Geometry: final body of the model. Coordinates: model frame, mm. A direction names the side the tool comes from. Coordinates: 2 decimals unless noted, no trailing zeros. Order: outer loops, then holes, each group sorted by start corner. A loop starts at its lowest first (then second) coordinate and runs counter-clockwise, first axis right, second up. Notation, with made-up numbers: (20, 72.25) -> (77, 72.25) arc R6 cw to (77, 77.25) -> close; hole circle Ø5 at (86.25, -0.75). An arc over 180 degrees is marked (long way). Answer in a Markdown table with one row per item. Add a question column.
1) Section query D-D on x = 7.5. Return the cut outline in (y, z).
2) Section query B-B on y = 29.5. Return the cut outline in (x, z).
3) Set-up query: faces 1 (the face through (12.7, 45, -43)), 2 (the face through (1, 13, 0)), 3 (the face through (-12.7, 45, -43)), 4 (the face through (1, 13, -101.6)). Return all of +Z, -Z, +X, -X, +Y, -Y with unobstructed straight access to the full face (end or side cutting, diameter ignored); none if empty.
4) Section query A-A on x = 22.5. Return the cut outline in (y, z).
5) Section query C-C on z = -19. Return the cut outline in (x, y), then the cut area to 3 significant figures.
6) Pull-direction query (Z, two-part tool) for faces 5 (the face through (-38.1, 32, -65)), 6 (the face through (-5.47, 127.15, -90.68)), 7 (the face through (3.72, 101.245, -119.34)); classes: +Z half, -Z half, draft (parallel to the pull), parting line (faces both ways), or undercut.
7) Contact query for flat-ended pins moving along their axis: P1, Ø10, axis at x = 25.5, y = 95, coming from the +Z side; P2, Ø10, axis at y = 84.5, z = -131, coming from the -X side; P3, Ø10, axis at x = -14.5, y = 14, coming from the -Z side. Output: stop coordinate, or through.
8) Ray query, line 1 (X direction, y = 38.5, z = -40); line 2 (Y direction, x = 24.5, z = -35); line 3 (X direction, y = 82, z = -121.5). Return the intervals inside material, ascending. Write a range as from..to.
```python
from build123d import *

# Parameters (mm, degrees)
BOSS_EXTRUDE1_DEPTH = 38.1
BOSS_EXTRUDE2_REACH = 114.341
SKETCH3_W           = 25.4
SKETCH3_H           = 88.161149917
SKETCH4_R           = 38.1
BOSS_EXTRUDE3_DEPTH = 76.2
SKETCH5_R           = 28.575
CUT_EXTRUDE1_DEPTH  = 76.2


with BuildPart() as part:
    # Sketch1 → Boss-Extrude1 (new body, symmetric)
    with BuildSketch(Plane(origin=(0, 0, 0), x_dir=(0, 0, -1), z_dir=(1, 0, 0))):
        Polygon((0, 0), (0, 25.4), (50.8, 25.4), (100.244555556, 80.313742191), (128.299578523, 55.052886048), (101.6, 25.4), (101.6, 0), align=None)
    extrude(amount=BOSS_EXTRUDE1_DEPTH, both=True)

    # Sketch3 → Boss-Extrude2 (add, up to next)
    with BuildSketch(Plane(origin=(0, 11.372488517, 12.630428071), x_dir=(1, 0, 0), z_dir=(0, 0.669130606, 0.743144825)), mode=Mode.PRIVATE) as boss_extrude2_sk1:
        with Locations((0, 62.956453526)):
            Rectangle(SKETCH3_W, SKETCH3_H)
    boss_extrude2_tool1 = extrude(boss_extrude2_sk1.sketch, amount=-BOSS_EXTRUDE2_REACH, mode=Mode.PRIVATE) - part.part
    add(boss_extrude2_tool1.solids().sort_by_distance((0, 58.158251, -29.495662))[0])

    # Sketch4 → Boss-Extrude3 (add)
    with BuildSketch(Plane(origin=(0, -39.149223768, -43.479617863), x_dir=(-1, 0, 0), z_dir=(0, -0.669130606, -0.743144825))):
        with Locations((0, 126.761442167)):
            Circle(SKETCH4_R)
    extrude(amount=-BOSS_EXTRUDE3_DEPTH)

    # Sketch5 → Cut-Extrude1 (cut)
    with BuildSketch(Plane(origin=(0, -39.149223768, -43.479617863), x_dir=(-1, 0, 0), z_dir=(0, -0.669130606, -0.743144825))):
        with Locations((0, 126.761442167)):
            Circle(SKETCH5_R)
    extrude(amount=-CUT_EXTRUDE1_DEPTH, mode=Mode.SUBTRACT)


solid = part.part
```
Result:
| question | item | result |
|---|---|---|
| 1 | outline | (0, -101.6) -> (25.4, -101.6) -> (34.56, -109.85) -> (85.55, -53.22) -> (78.28, -46.68) -> (77.81, -47.19) -> (25.4, 0) -> (0, 0) -> close; (75.54, -146.75) -> (82.81, -153.29) -> (133.8, -96.67) -> (126.53, -90.12) -> close |
| 2 | outline | (-38.1, -105.29) -> (38.1, -105.29) -> (38.1, -54.49) -> (12.7, -54.49) -> (12.7, -3.69) -> (-12.7, -3.69) -> (-12.7, -54.49) -> (-38.1, -54.49) -> close |
| 3 | face 1 | +Z, +X |
| 3 | face 2 | +Z, +X, -X, +Y, -Y |
| 3 | face 3 | +Z, -X |
| 3 | face 4 | -Z, +X, -X, -Y |
| 4 | outline | (0, -101.6) -> (25.4, -101.6) -> (41.96, -116.51) -> (92.95, -59.89) -> (83.19, -51.1) -> (57.46, -79.67) -> (25.4, -50.8) -> (25.4, 0) -> (0, 0) -> close; (68.14, -140.09) -> (77.9, -148.87) -> (128.89, -92.25) -> (119.13, -83.46) -> close |
| 5 | outline | (-38.1, 0) -> (38.1, 0) -> (38.1, 25.4) -> (12.7, 25.4) -> (12.7, 46.5) -> (-12.7, 46.5) -> (-12.7, 25.4) -> (-38.1, 25.4) -> close |
| 5 | area | 2,470 mm2 |
| 6 | face 5 | draft |
| 6 | face 6 | +Z half |
| 6 | face 7 | undercut |
| 7 | P1 | z = -57.23 |
| 7 | P2 | x = -33.2 |
| 7 | P3 | z = -101.6 |
| 8 | line 1 | -12.7..12.7 |
| 8 | line 2 | 0..25.4 |
| 8 | line 3 | -34.82..-24.02, 24.02..34.82 |
